Answer from the drawing. Dimensions are ordinates in mm from the lowest x, y and z of the part. A direction names the side the tool comes from. Round coordinates to 2 decimals unless told otherwise and drop trailing zeros. Loops run counter-clockwise (first coordinate to the right, second up) from the corner with the lowest first, then second, coordinate; pieces in that order, holes last.
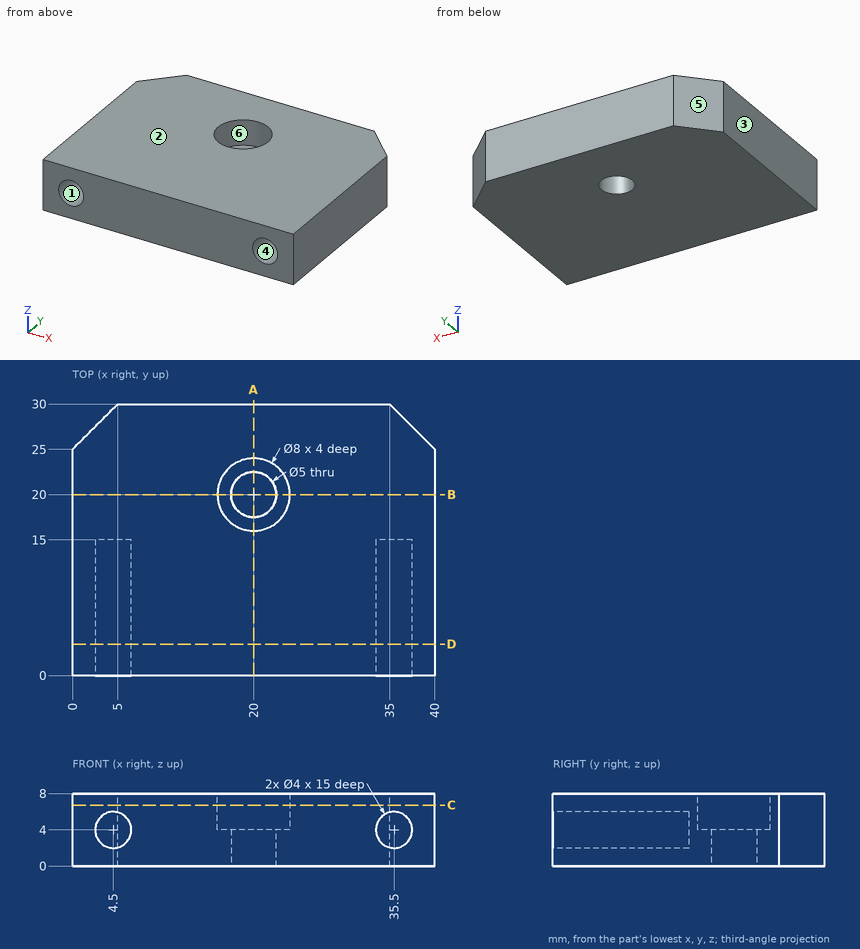
1. Find section D-D (y = 3.5). Write down the section's boundary in (x, z).
Answer key:
outline: (0, 0) - (40, 0) - (40, 8) - (0, 8) - close; hole circle Ø4 at (4.5, 4); hole circle Ø4 at (35.5, 4)
2. Consider probe 1 along Z at (x, y) = (35.5, 3.75); probe 2 along Y at (x, z) = (20, 7.1); probe 3 along Y at (x, z) = (20, 2.45). Determine where each line is inside the solid, lowest interval first.
Answer key:
probe 1: z = 0 to 2, 6 to 8
probe 2: y = 0 to 16, 24 to 30
probe 3: y = 0 to 17.5, 22.5 to 30
3. Which of the six approach directions +Z, -Z, +X, -X, +Y, -Y give full straight-line access (tool end or side, diameter ignored) to the marked faces 4, 5 and 6?
Answer key:
face 4: -Y
face 5: +Z, -Z, -X, +Y
face 6: +Z
4. Determine the mould class of the marked faces 1, 2 and 3 for opening direction Z: +Z half, -Z half, draft (parallel to the pull), parting line (faces both ways), or undercut.
Answer key:
face 1: undercut
face 2: +Z half
face 3: draft
5. Find section A-A (x = 20). Write down the section's boundary in (y, z), then the cut area to 3 significant figures.
Answer key:
outline: (0, 0) - (17.5, 0) - (17.5, 4) - (16, 4) - (16, 8) - (0, 8) - close; (22.5, 0) - (30, 0) - (30, 8) - (24, 8) - (24, 4) - (22.5, 4) - close
area: 188 mm2
6. Find section C-C (z = 6.75). Write down the section's boundary in (x, y), then the cut area to 3 significant figures.
Answer key:
outline: (0, 0) - (40, 0) - (40, 25) - (35, 30) - (5, 30) - (0, 25) - close; hole circle Ø8 at (20, 20)
area: 1,120 mm2
7. Find section B-B (y = 20). Write down the section's boundary in (x, z), then the cut area to 3 significant figures.
Answer key:
outline: (0, 0) - (17.5, 0) - (17.5, 4) - (16, 4) - (16, 8) - (0, 8) - close; (22.5, 0) - (40, 0) - (40, 8) - (24, 8) - (24, 4) - (22.5, 4) - close
area: 268 mm2
8. Given pin 1 (1.2 mm diameter, centred on x = 34.5, z = 3.5, fed in from -Y); pin 2 (6.5 mm diameter, centred on x = 19.5, y = 19.5, fed in from +Z), each flat-ended and moving along its own axis, determine where each tip first touches the part or whether it passes through.
Answer key:
pin 1: stops at y = 15
pin 2: stops at z = 4
